```python
from build123d import *

# Parameters (mm, degrees)
SKETCH1_W           = 89.4
SKETCH1_H           = 76.4
BOSS_EXTRUDE1_DEPTH = 6
SKETCH1_5_W         = 85.4
SKETCH1_5_H         = 72.4
CUT_EXTRUDE2_DEPTH  = 1.6
CUT_EXTRUDE3_DEPTH  = 3
SKETCH1_7_R         = 1.45
CUT_EXTRUDE4_DEPTH  = 82.868794295
FILLET1_R           = 1
SKETCH2_R           = 3.5
CUT_EXTRUDE5_DEPTH  = 3


with BuildPart() as part:
    # Sketch1 → Boss-Extrude1 (new body)
    with BuildSketch(Plane(origin=(0, 0, 0), x_dir=(1, 0, 0), z_dir=(0, 1, 0))):
        with Locations((-24.890531337, 4.504302213)):
            Rectangle(SKETCH1_W, SKETCH1_H)
    extrude(amount=-BOSS_EXTRUDE1_DEPTH)

    # Sketch1_5 → Cut-Extrude2 (cut)
    with BuildSketch(Plane(origin=(0, 0, 0), x_dir=(1, 0, 0), z_dir=(0, 1, 0))):
        with Locations((-24.890531337, 4.504302213)):
            Rectangle(SKETCH1_5_W, SKETCH1_5_H)
    extrude(amount=-CUT_EXTRUDE2_DEPTH, mode=Mode.SUBTRACT)

    # Sketch1_6 → Cut-Extrude3 (cut)
    with BuildSketch(Plane(origin=(0, 0, 0), x_dir=(1, 0, 0), z_dir=(0, 1, 0))):
        Polygon((-47.775836727, -21.495697787), (-65.590531337, -21.495697787), (-65.590531337, 29.568169386), (-56.990531337, 29.568169386), (-56.990531337, 38.704302213), (8.309468663, 38.704302213), (8.309468663, 29.504302213), (15.809468663, 29.504302213), (15.809468663, -22.495697787), (8.609468663, -22.495697787), (8.609468663, -28.695697787), (-47.775836727, -28.695697787), align=None)
    extrude(amount=-CUT_EXTRUDE3_DEPTH, mode=Mode.SUBTRACT)

    # Sketch1_7 → Cut-Extrude4 (cut, through all)
    with BuildSketch(Plane(origin=(0, 0, 0), x_dir=(1, 0, 0), z_dir=(0, 1, 0))):
        with Locations(Location((13.609468663, 36.504302213, 0), (0, 0, 270))):
            Circle(SKETCH1_7_R)
        with Locations(Location((-63.775836727, -27.495697787, 0), (0, 0, 270))):
            Circle(SKETCH1_7_R)
        with Locations(Location((-63.390531337, 36.504302213, 0), (0, 0, 270))):
            Circle(SKETCH1_7_R)
        with Locations(Location((13.609468663, -27.495697787, 0), (0, 0, 270))):
            Circle(SKETCH1_7_R)
    extrude(amount=-CUT_EXTRUDE4_DEPTH, mode=Mode.SUBTRACT)

    # Fillet1
    fillet1_edges = [part.edges().sort_by_distance(p)[0] for p in [
        (-69.590531337, -3, -42.704302213),
        (19.809468663, -3, -42.704302213),
        (19.809468663, -3, 33.695697787),
        (-69.590531337, -3, 33.695697787),
    ]]
    fillet(fillet1_edges, radius=FILLET1_R)

    # Sketch2 → Cut-Extrude5 (cut)
    with BuildSketch(Plane.XZ.offset(6)):
        with Locations(Location((-63.775836727, 27.495697787, 0), (0, 0, 270))):
            Circle(SKETCH2_R)
        with Locations(Location((13.609468663, 27.495697787, 0), (0, 0, 270))):
            Circle(SKETCH2_R)
        with Locations(Location((13.609468663, -36.504302213, 0), (0, 0, 270))):
            Circle(SKETCH2_R)
        with Locations(Location((-63.390531337, -36.504302213, 0), (0, 0, 270))):
            Circle(SKETCH2_R)
    extrude(amount=-CUT_EXTRUDE5_DEPTH, mode=Mode.SUBTRACT)


solid = part.part
```
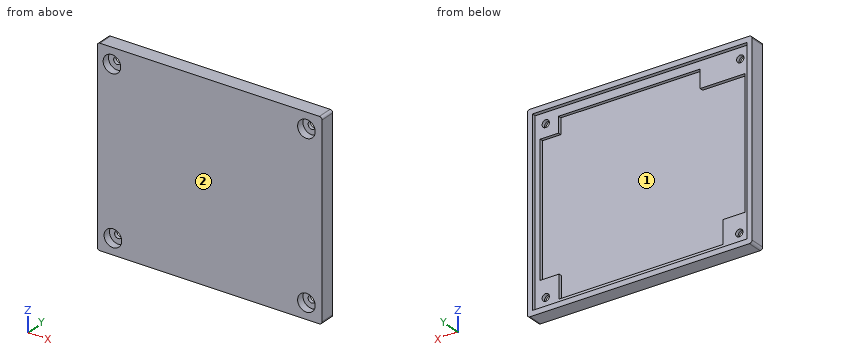
Model file for the job. Use its own axes, mm. Face numbers are marked on the shaded views. A direction names the side the tool comes from. Give positions to 0.01 mm unless a question says otherwise; leave off trailing zeros. Loops run counter-clockwise (first coordinate to the right, second up) from the corner with the lowest first, then second, coordinate; pieces in that order, holes last. Notation, with made-up numbers: (16, 70) - (53, 70) arc R23 ccw to (53, 95) - close; hole circle Ø1 at (45, -30.75). An arc over 180 degrees is marked (long way). One line per item, written item: value. Start each with the question number.
1. Probe L1, parallel to X at y = -2.2, z = -4.5; L2, parallel to Z at x = -41.5, y = -2.7; L3, parallel to X at y = -4.2, z = 27.5. List the from-to ranges inside material, lowest first. Write a range as from..to.
2. Slice it at B-B (z = -36). List the corners of the cut face in (x, y), plus the area to 3 significant figures.
3. Slice it at C-C (y = -4.7). List the corners of the cut face in (x, z), plus the area to 3 significant figures.
4. Slice it at A-A (z = -17). List the corners of the cut face in (x, y), plus the area to 3 significant figures.
5. Pin check, flat tips, straight feed: pin 1 (2 mm diameter, centred on x = 15, z = 27, fed in from -Y); pin 2 (1.5 mm diameter, centred on x = -56, z = 10, fed in from +Y); pin 3 (6.5 mm diameter, centred on x = -63.78, z = 27.5, fed in from +Y). Stop position of each tip, or through.
6. Which spindle directions (+Z, -Z, +X, -X, +Y, -Y) get a long thin tool onto all of the face, cutting with end or side? Do the marked faces 1 and 2. Say none if no direction does.
7. Slice it at D-D (x = 3). List the corners of the cut face in (y, z), plus the area to 3 significant figures.
Solution:
1. L1: x = -69.59..-65.59, 15.81..19.81
1. L2: z = -42.7..-38.7, 28.7..33.7
1. L3: x = -69.59..-67.28, -60.28..10.11, 17.11..19.81
2. outline: (-69.59, -6) - (-66.85, -6) - (-66.85, -3) - (-64.75, -3) - (-64.75, -1.6) - (-67.59, -1.6) - (-67.59, 0) - (-69.59, 0) - close; (-62.03, -3) - (-59.93, -3) - (-59.93, -6) - (10.15, -6) - (10.15, -3) - (12.25, -3) - (12.25, -1.6) - (8.31, -1.6) - (8.31, -3) - (-56.99, -3) - (-56.99, -1.6) - (-62.03, -1.6) - close; (14.97, -3) - (17.07, -3) - (17.07, -6) - (19.81, -6) - (19.81, 0) - (17.81, 0) - (17.81, -1.6) - (14.97, -1.6) - close
2. area: 259 mm^2
3. outline: (-69.59, -41.7) arc R1 ccw to (-68.59, -42.7) - (18.81, -42.7) arc R1 ccw to (19.81, -41.7) - (19.81, 32.7) arc R1 ccw to (18.81, 33.7) - (-68.59, 33.7) arc R1 ccw to (-69.59, 32.7) - close; hole circle Ø7 at (-63.78, 27.5); hole circle Ø7 at (-63.39, -36.5); hole circle Ø7 at (13.61, -36.5); hole circle Ø7 at (13.61, 27.5)
3. area: 6,680 mm^2
4. outline: (-69.59, -6) - (19.81, -6) - (19.81, 0) - (17.81, 0) - (17.81, -1.6) - (15.81, -1.6) - (15.81, -3) - (-65.59, -3) - (-65.59, -1.6) - (-67.59, -1.6) - (-67.59, 0) - (-69.59, 0) - close
4. area: 286 mm^2
5. pin 1: stops at y = -3
5. pin 2: stops at y = -3
5. pin 3: stops at y = -1.6
6. face 1: +Y
6. face 2: +Z, -Z, +X, -X, -Y
7. outline: (-6, -42.7) - (0, -42.7) - (0, -40.7) - (-1.6, -40.7) - (-1.6, -38.7) - (-3, -38.7) - (-3, 28.7) - (-1.6, 28.7) - (-1.6, 31.7) - (0, 31.7) - (0, 33.7) - (-6, 33.7) - close
7. area: 248 mm^2
